Input: dimensioned drawing with shaded views. Units: mm. Origin: part minimum x, y, z. A direction names the side the tool comes from. Round coordinates to 2 decimals unless told otherwise and drop trailing zeros. Order: outer loops, then holes, each group sorted by start corner. A loop starts at its lowest first (then second) coordinate and runs counter-clockwise, first axis right, second up. Notation, with made-up numbers: (-26.5, 8.5) - (2.5, 8.5) arc R33 cw to (2.5, 36.5) - close; hole circle Ø5 at (89, 14.25). An arc over 180 degrees is marked (long way). Return JSON: item names as keys, results as strings. Group by question number.
1) Section D-D, the plane z = 3.5. Return loops of the section in (x, y), plus the area to 3 significant figures.
2) Section C-C, the plane y = 3. Return loops of the section in (x, z).
3) Contact query for flat-ended pins moving along their axis: P1, Ø3, axis at x = 24, y = 3.56, coming from the -Z side; P2, Ø9.5, axis at x = 24, y = 18.56, coming from the +Z side; P3, Ø2.5, axis at x = 20, z = 11.5, coming from the -Y side; P4, Ø3, axis at y = 17.5, z = 2, coming from the +X side. Output: stop coordinate, or through.
4) Mould query, pull axis X, two halves, no side actions, for the marked faces 3, 4 and 5. Classes: pulls with the +X half, pulls with the -X half, needs draft (parallel to the pull), parting line crosses it, or undercut.
5) Section A-A, the plane z = 12. Give the number of separate pieces and of enclosed holes in the cut face, plus the area to 3 significant figures.
6) Ray query, line 1 (Y direction, x = 24, z = 0.75) (1 decimal); line 2 (Y direction, x = 24, z = 3.55); line 3 (X direction, y = 2, z = 3.5). Return the intervals inside material, ascending. Write a range as from..to.
7) Section B-B, the plane x = 29.5. Return loops of the section in (y, z) (1 decimal), plus the area to 3 significant figures.
8) Access query for the marked faces 1 and 2. Directions: +Z, -Z, +X, -X, +Y, -Y. A direction counts if a zero-diameter tool reaches every point of the face in a straight line with its end or side. Return the directions, or none.
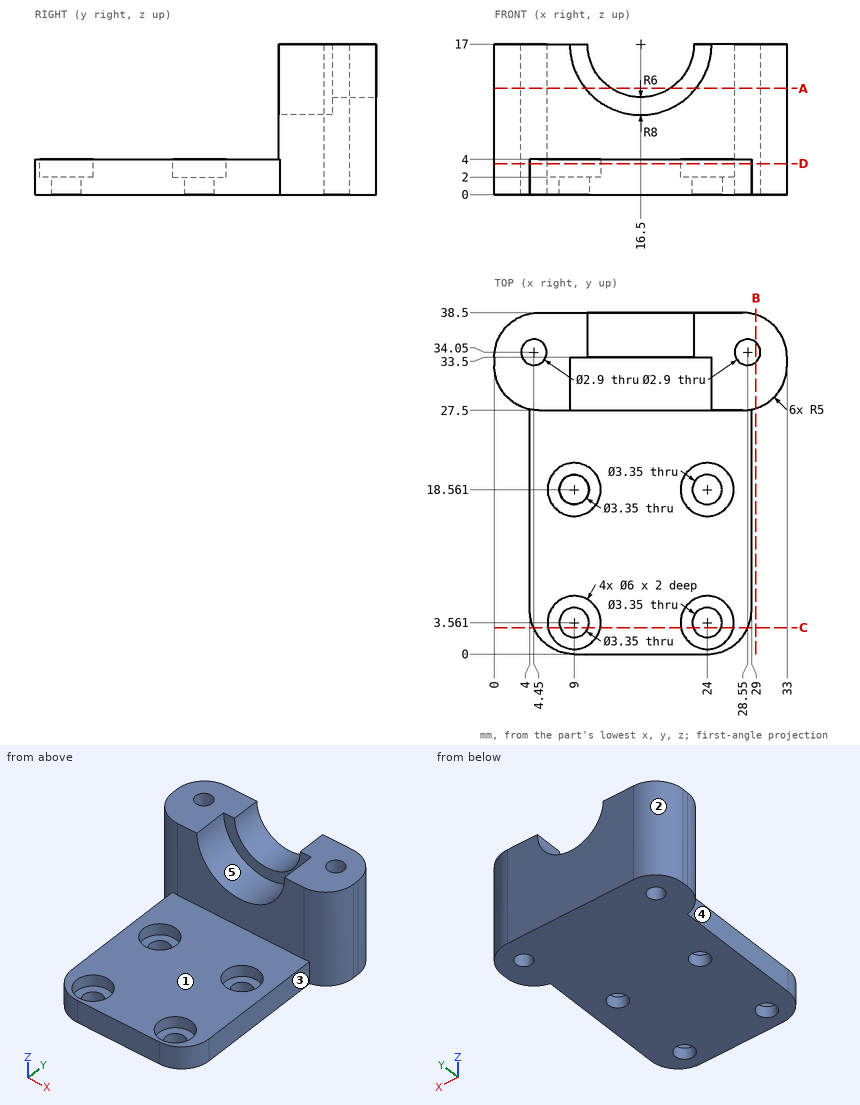
Geometry check:
{
 "1": {"outline": "(0, 32.5) arc R5 ccw to (4, 27.6) - (4, 5) arc R5 ccw to (9, 0) - (24, 0) arc R5 ccw to (29, 5) - (29, 27.6) arc R5 ccw to (33, 32.5) - (33, 33.5) arc R5 ccw to (28, 38.5) - (5, 38.5) arc R5 ccw to (0, 33.5) - close; hole circle Ø2.9 at (4.45, 34.05); hole circle Ø6 at (9, 3.56); hole circle Ø6 at (9, 18.56); hole circle Ø6 at (24, 3.56); hole circle Ø6 at (24, 18.56); hole circle Ø2.9 at (28.55, 34.05)", "area": "892 mm2"},
 "2": {"outline": "(4.42, 0) - (7.42, 0) - (7.42, 2) - (6.05, 2) - (6.05, 4) - (4.42, 4) - close; (10.58, 0) - (22.42, 0) - (22.42, 2) - (21.05, 2) - (21.05, 4) - (11.95, 4) - (11.95, 2) - (10.58, 2) - close; (25.58, 0) - (28.58, 0) - (28.58, 4) - (26.95, 4) - (26.95, 2) - (25.58, 2) - close"},
 "3": {"P1": "through", "P2": "z = 4", "P3": "y = 33.5", "P4": "x = 29"},
 "4": {"face 3": "pulls with the +X half", "face 4": "pulls with the -X half", "face 5": "undercut"},
 "5": {"separate pieces": "2", "enclosed holes": "2", "area": "220 mm2"},
 "6": {"line 1": "0..1.9, 5.2..16.9, 20.2..38.5", "line 2": "0..0.56, 6.56..15.56, 21.56..38.5", "line 3": "5..6.44, 11.56..21.44, 26.56..28"},
 "7": {"outline": "(27.7, 0) - (33, 0) - (33, 17) - (27.7, 17) - close; (35.1, 0) - (38.3, 0) - (38.3, 17) - (35.1, 17) - close", "area": "142 mm2"},
 "8": {"face 1": "+Z, +X, -X, -Y", "face 2": "+Z, -Z, -X, +Y"}
}
